Read the model definition and answer for the solid it produces. Units are mm, in the model's axes. A direction names the side the tool comes from. Coordinates: 2 decimals unless noted, no trailing zeros. Loops run counter-clockwise (first coordinate to the right, second up) from the corner with the lowest first, then second, coordinate; pieces in that order, holes last. Notation, with made-up numbers: (29.5, -38.75) -> (37.5, -38.75) arc R23 ccw to (37.5, -10.75) -> close; hole circle Ø7 at (-34.5, -6). An arc over 180 degrees is marked (long way). Answer as CSV lines item,"result".
```python
from build123d import *

# Parameters (mm, degrees)
BOSS_EXTRUDE1_START = 1.27
BOSS_EXTRUDE1_DEPTH = 1.27


with BuildPart() as part:
    # Sweep1: sweep along a path in Sketch2
    with BuildLine(Plane(origin=(0, 428.625, 0), x_dir=(1, 0, 0), z_dir=(0, 1, 0))) as sweep1_path:
        Line((-249.2375, -230.1875), (249.2375, -230.1875))
        ThreePointArc((249.2375, -230.1875), (267.198012242, -222.748012242), (274.6375, -204.7875))
        Line((274.6375, -204.7875), (274.6375, 204.7875))
        ThreePointArc((274.6375, 204.7875), (267.198012242, 222.748012242), (249.2375, 230.1875))
        Line((249.2375, 230.1875), (-249.2375, 230.1875))
        ThreePointArc((-249.2375, 230.1875), (-267.198012242, 222.748012242), (-274.6375, 204.7875))
        Line((-274.6375, 204.7875), (-274.6375, -204.7875))
        ThreePointArc((-274.6375, -204.7875), (-267.198012242, -222.748012242), (-249.2375, -230.1875))
    # Sketch3 → Sweep1 (sweep)
    with BuildSketch(Plane.XY):
        with BuildLine():
            Line((-274.6375, 428.625), (-275.02653488, 431.318318399))
            ThreePointArc((-275.02653488, 431.318318399), (-275.452129987, 432.096831513), (-276.283489893, 432.406758231))
            Line((-276.283489893, 432.406758231), (-279.341510107, 432.406758231))
            ThreePointArc((-279.341510107, 432.406758231), (-280.172870013, 432.096831513), (-280.59846512, 431.318318399))
            Line((-280.59846512, 431.318318399), (-280.9875, 428.625))
            Line((-280.9875, 428.625), (-282.821944444, 415.925))
            Line((-282.821944444, 415.925), (-284.078899458, 416.106560169))
            Line((-284.078899458, 416.106560169), (-282.244455013, 428.806560169))
            Line((-282.244455013, 428.806560169), (-281.855420133, 431.499878568))
            ThreePointArc((-281.855420133, 431.499878568), (-281.004229918, 433.056904795), (-279.341510107, 433.676758231))
            Line((-279.341510107, 433.676758231), (-276.283489893, 433.676758231))
            ThreePointArc((-276.283489893, 433.676758231), (-274.620770082, 433.056904795), (-273.769579867, 431.499878568))
            Line((-273.769579867, 431.499878568), (-273.537764074, 429.895))
            Line((-273.537764074, 429.895), (-273.537764074, 428.625))
            Line((-273.537764074, 428.625), (-274.6375, 428.625))
        make_face()
    sweep(path=sweep1_path.line)

    # Sketch6 → Boss-Extrude1 (add)
    with BuildSketch(Plane(origin=(0, 428.625, 0), x_dir=(1, 0, 0), z_dir=(0, 1, 0)).offset(BOSS_EXTRUDE1_START)):
        with BuildLine():
            Line((249.2375, 229.087764074), (-249.2375, 229.087764074))
            ThreePointArc((-249.2375, 229.087764074), (-266.420381511, 221.970381511), (-273.537764074, 204.7875))
            Line((-273.537764074, 204.7875), (-273.537764074, 0))
            Line((-273.537764074, 0), (-273.537764074, -204.7875))
            ThreePointArc((-273.537764074, -204.7875), (-266.420381511, -221.970381511), (-249.2375, -229.087764074))
            Line((-249.2375, -229.087764074), (249.2375, -229.087764074))
            ThreePointArc((249.2375, -229.087764074), (266.420381511, -221.970381511), (273.537764074, -204.7875))
            Line((273.537764074, -204.7875), (273.537764074, 204.7875))
            ThreePointArc((273.537764074, 204.7875), (266.420381511, 221.970381511), (249.2375, 229.087764074))
        make_face()
    extrude(amount=-BOSS_EXTRUDE1_DEPTH)


solid = part.part
```
Q1. For faces 4 (the face through (273.388, 415.954, -228.413)), 5 (the face through (4, 428.625, 3)), 6 (the face through (-266.655, 430.352, 221.827)), determine the directions among +Z, -Z, +X, -X, +Y, -Y from which every point of the face is accessible in a straight line to the end or side of a thin tool.
Results:
face 4,"-Z, +X, -Y"
face 5,"-Y"
face 6,"+Y"
Q2. A cutting plane is placed at C-C, the plane y = 421.75. Write down the section's boundary in (x, z), and give its area (3 significant figures).
Results:
outline,"(-283.26, -204.79) arc R34.03 ccw to (-249.24, -238.81) -> (249.24, -238.81) arc R34.03 ccw to (283.26, -204.79) -> (283.26, 204.79) arc R34.03 ccw to (249.24, 238.81) -> (-249.24, 238.81) arc R34.03 ccw to (-283.26, 204.79) -> close; hole (-281.98, -204.79) arc R32.74 ccw to (-249.24, -237.53) -> (249.24, -237.53) arc R32.74 ccw to (281.98, -204.79) -> (281.98, 204.79) arc R32.74 ccw to (249.24, 237.53) -> (-249.24, 237.53) arc R32.74 ccw to (-281.98, 204.79) -> close"
area,"2,600 mm²"
Q3. For a pull along X with two mould halves and no side action, classify faces 1 (the face through (272.863, 415.954, 228.938)), 2 (the face through (-267.103, 429.654, -223.051)), 3 (the face through (-273.388, 415.954, 228.413)) as pulls with the +X half, pulls with the -X half, needs draft (parallel to the pull), parting line crosses it, or undercut.
Results:
face 1,"pulls with the +X half"
face 2,"undercut"
face 3,"pulls with the -X half"
Q4. A cutting plane is placed at B-B, the plane x = 176.5. Write down the section's boundary in (y, z) (1 decimal), and give its area (3 significant figures).
Results:
outline,"(415.9, -238.4) -> (416.1, -239.6) -> (431.5, -237.4) arc R2.5 ccw to (433.7, -234.9) -> (433.7, -231.8) arc R2.5 ccw to (431.5, -229.3) -> (429.9, -229.1) -> (429.9, 229.1) -> (431.5, 229.3) arc R2.5 ccw to (433.7, 231.8) -> (433.7, 234.9) arc R2.5 ccw to (431.5, 237.4) -> (416.1, 239.6) -> (415.9, 238.4) -> (431.3, 236.1) arc R1.3 cw to (432.4, 234.9) -> (432.4, 231.8) arc R1.3 cw to (431.3, 230.6) -> (428.6, 230.2) -> (428.6, -230.2) -> (431.3, -230.6) arc R1.3 cw to (432.4, -231.8) -> (432.4, -234.9) arc R1.3 cw to (431.3, -236.1) -> close"
area,"650 mm²"
Q5. A cutting plane is placed at A-A, the plane z = -66.5. Write down the section's boundary in (x, y) (1 decimal).
Results:
outline,"(-284.1, 416.1) -> (-282.8, 415.9) -> (-280.6, 431.3) arc R1.3 cw to (-279.3, 432.4) -> (-276.3, 432.4) arc R1.3 cw to (-275, 431.3) -> (-274.6, 428.6) -> (274.6, 428.6) -> (275, 431.3) arc R1.3 cw to (276.3, 432.4) -> (279.3, 432.4) arc R1.3 cw to (280.6, 431.3) -> (282.8, 415.9) -> (284.1, 416.1) -> (281.9, 431.5) arc R2.5 ccw to (279.3, 433.7) -> (276.3, 433.7) arc R2.5 ccw to (273.8, 431.5) -> (273.5, 429.9) -> (-273.5, 429.9) -> (-273.8, 431.5) arc R2.5 ccw to (-276.3, 433.7) -> (-279.3, 433.7) arc R2.5 ccw to (-281.9, 431.5) -> close"
Q6. Given pin 1 Ø4 at (y, z) = (419.5, -127) entering from +X; pin 2 Ø1.5 at (x, z) = (-72.5, -34.5) entering from -Y (3 decimals); pin 3 Ø4 at (x, y) = (-161.5, 418.5) entering from -Z, each flat-ended and moving along its own axis, determine where each tip first touches the part or whether it passes through.
Results:
pin 1,"stops at x = 283.88"
pin 2,"stops at y = 428.625"
pin 3,"stops at z = -239.57"
Q7. Find the intervals of material crossed by probe 1 along X at (y, z) = (431, 45.5); probe 2 along Z at (x, y) = (-179, 428.75); probe 3 along X at (y, z) = (430.5, -135.5), in increasing order. Write a range as [from, to].
Results:
probe 1,"x = [-281.93, -280.64], [-274.98, -273.7], [273.7, 274.98], [280.64, 281.93]"
probe 2,"z = [-237.8, -236.52], [-230.21, 230.21], [236.52, 237.8]"
probe 3,"x = [-282, -280.72], [-274.91, -273.63], [273.63, 274.91], [280.72, 282]"
